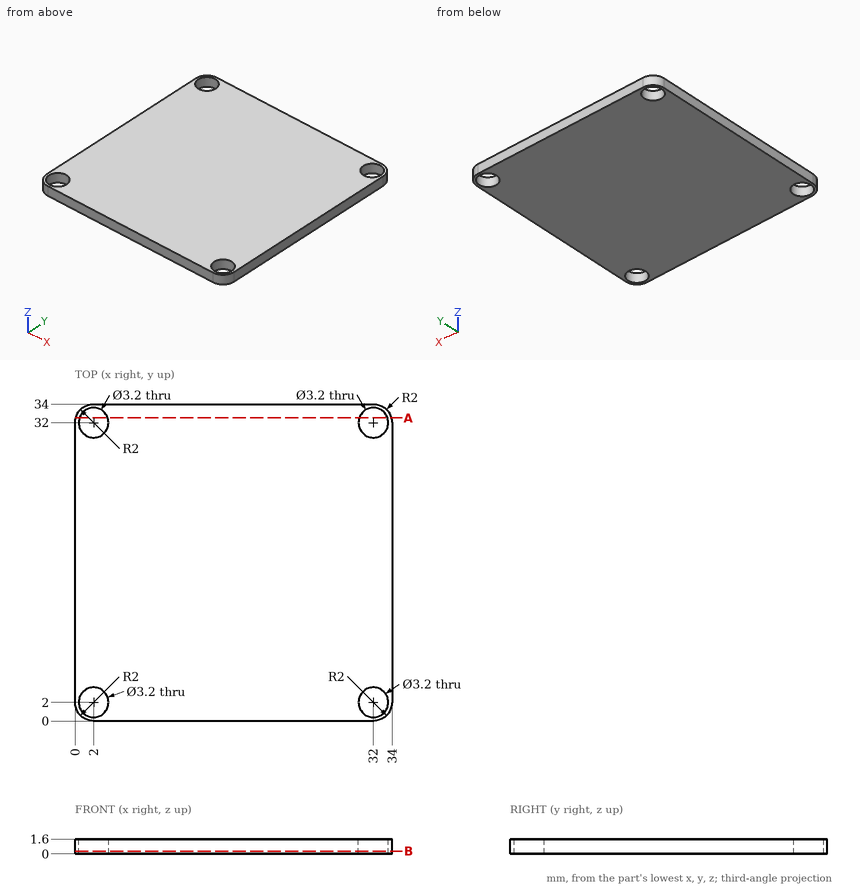
Could you check a few things on this drawing? It's one solid part, dimensions in mm from its lowest x, y, z. Coordinates: 2 decimals unless noted, no trailing zeros. Write each loop counter-clockwise with the first axis right and the second up, starting at its lowest first coordinate (ties: lowest second). Pieces come first, ordered by that corner, then holes.
1) If we section it at A-A (y = 32.5): List the corners of the cut face in (x, z) for me.
Filled in:
outline: (0.06, 0) - (0.48, 0) - (0.48, 1.6) - (0.06, 1.6) - close; (3.52, 0) - (30.48, 0) - (30.48, 1.6) - (3.52, 1.6) - close; (33.52, 0) - (33.94, 0) - (33.94, 1.6) - (33.52, 1.6) - close
2) If I drill on line 1 (Y direction, x = 32, z = 0.65), over which ranges is the centre line in solid material (lowest first)?
Filled in:
line 1: y = 0 to 0.4, 3.6 to 30.4, 33.6 to 34
3) If we section it at B-B (z = 0.3): List the corners of the cut face in (x, y) for me.
Filled in:
outline: (0, 2) arc R2 ccw to (2, 0) - (32, 0) arc R2 ccw to (34, 2) - (34, 32) arc R2 ccw to (32, 34) - (2, 34) arc R2 ccw to (0, 32) - close; hole circle Ø3.2 at (2, 2); hole circle Ø3.2 at (2, 32); hole circle Ø3.2 at (32, 2); hole circle Ø3.2 at (32, 32)
4) I'm going to push flat-ended pins straight in: pin 1 (1.5 mm diameter, centred on x = 23, y = 15.5, fed in from -Z); pin 2 (2.5 mm diameter, centred on x = 32, y = 2, fed in from -Z). Where does each tip first touch, or does it pass through?
Filled in:
pin 1: stops at z = 0
pin 2: passes through
